from build123d import *

# Parameters (mm, degrees)
SKETCH_1_W               = 40
SKETCH_1_H               = 30
EXTRUDE_1_DEPTH          = 125
SKETCH_2_W               = 38
SKETCH_2_H               = 28
CUT_EXTRUDE_1_DEPTH      = 126
CUT_EXTRUDE_1_DEPTH_BACK = 126
SKETCH_3_R               = 2.025
CUT_EXTRUDE_2_DEPTH      = 1
CUT_EXTRUDE_2_DEPTH_BACK = 31
SKETCH_4_R               = 2.025
CUT_EXTRUDE_3_DEPTH      = 1
CUT_EXTRUDE_3_DEPTH_BACK = 31
CUT_EXTRUDE_4_DEPTH      = 1
CUT_EXTRUDE_4_DEPTH_BACK = 41
CUT_EXTRUDE_5_DEPTH      = 1
CUT_EXTRUDE_5_DEPTH_BACK = 31
CUT_EXTRUDE_6_DEPTH      = 1
CUT_EXTRUDE_6_DEPTH_BACK = 41


with BuildPart() as part:
    # 草图1 → 凸台-拉伸1 (new body, symmetric)
    with BuildSketch(Plane(origin=(0, 0, 0), x_dir=(1, 0, 0), z_dir=(0, 1, 0))):
        Rectangle(SKETCH_1_W, SKETCH_1_H)
    extrude(amount=EXTRUDE_1_DEPTH, both=True)

    # 草图2 → 切除-拉伸1 (cut, two sides)
    with BuildSketch(Plane(origin=(0, 0, 0), x_dir=(1, 0, 0), z_dir=(0, 1, 0))) as cut_extrude_1_sk:
        Rectangle(SKETCH_2_W, SKETCH_2_H)
    extrude(amount=CUT_EXTRUDE_1_DEPTH, mode=Mode.SUBTRACT)
    extrude(cut_extrude_1_sk.sketch, amount=-CUT_EXTRUDE_1_DEPTH_BACK, mode=Mode.SUBTRACT)

    # 草图3 → 切除-拉伸2 (cut, two sides)
    with BuildSketch(Plane.XY.offset(15)) as cut_extrude_2_sk:
        with Locations((0, -62.433034374)):
            Circle(SKETCH_3_R)
        with Locations((0, -93.433034374)):
            Circle(SKETCH_3_R)
        with Locations((0, -121)):
            Circle(SKETCH_3_R)
    extrude(amount=CUT_EXTRUDE_2_DEPTH, mode=Mode.SUBTRACT)
    extrude(cut_extrude_2_sk.sketch, amount=-CUT_EXTRUDE_2_DEPTH_BACK, mode=Mode.SUBTRACT)

    # 草图4 → 切除-拉伸3 (cut, two sides)
    with BuildSketch(Plane(origin=(0, 0, -15), x_dir=(-1, 0, 0), z_dir=(0, 0, -1))) as cut_extrude_3_sk:
        with Locations((0, 120)):
            Circle(SKETCH_4_R)
        with Locations((12.5, 95)):
            Circle(SKETCH_4_R)
        with Locations((-12.5, 95)):
            Circle(SKETCH_4_R)
    extrude(amount=CUT_EXTRUDE_3_DEPTH, mode=Mode.SUBTRACT)
    extrude(cut_extrude_3_sk.sketch, amount=-CUT_EXTRUDE_3_DEPTH_BACK, mode=Mode.SUBTRACT)

    # 草图5 → 切除-拉伸4 (cut, two sides)
    with BuildSketch(Plane(origin=(20, 0, 0), x_dir=(0, 0, -1), z_dir=(1, 0, 0))) as cut_extrude_4_sk:
        with BuildLine():
            Line((-8, -100), (-8, -80))
            ThreePointArc((-8, -80), (0, -72), (8, -80))
            Line((8, -80), (8, -100))
            ThreePointArc((8, -100), (0, -108), (-8, -100))
        make_face()
    extrude(amount=CUT_EXTRUDE_4_DEPTH, mode=Mode.SUBTRACT)
    extrude(cut_extrude_4_sk.sketch, amount=-CUT_EXTRUDE_4_DEPTH_BACK, mode=Mode.SUBTRACT)

    # 草图6 → 切除-拉伸5 (cut, two sides)
    with BuildSketch(Plane(origin=(0, 0, -15), x_dir=(-1, 0, 0), z_dir=(0, 0, -1))) as cut_extrude_5_sk:
        with BuildLine():
            Line((-5, 115.5), (5, 115.5))
            ThreePointArc((5, 115.5), (13, 107.5), (5, 99.5))
            Line((5, 99.5), (-5, 99.5))
            ThreePointArc((-5, 99.5), (-13, 107.5), (-5, 115.5))
        make_face()
    extrude(amount=CUT_EXTRUDE_5_DEPTH, mode=Mode.SUBTRACT)
    extrude(cut_extrude_5_sk.sketch, amount=-CUT_EXTRUDE_5_DEPTH_BACK, mode=Mode.SUBTRACT)

    # 草图7 → 切除-拉伸6 (cut, two sides)
    with BuildSketch(Plane(origin=(20, 0, 0), x_dir=(0, 0, -1), z_dir=(1, 0, 0))) as cut_extrude_6_sk:
        with BuildLine():
            Line((-6, 45), (-6, 75))
            ThreePointArc((-6, 75), (0, 81), (6, 75))
            Line((6, 75), (6, 45))
            ThreePointArc((6, 45), (0, 39), (-6, 45))
        make_face()
        with BuildLine():
            Line((-6, -30), (-6, 0))
            ThreePointArc((-6, 0), (0, 6), (6, 0))
            Line((6, 0), (6, -30))
            ThreePointArc((6, -30), (0, -36), (-6, -30))
        make_face()
    extrude(amount=CUT_EXTRUDE_6_DEPTH, mode=Mode.SUBTRACT)
    extrude(cut_extrude_6_sk.sketch, amount=-CUT_EXTRUDE_6_DEPTH_BACK, mode=Mode.SUBTRACT)


solid = part.part
Can you work these out from the model? Positions are in its coordinate system, mm. A direction names the side the tool comes from. Give positions to 0.01 mm unless a question says otherwise; leave off trailing zeros. Order: outer loops, then holes, each group sorted by start corner. A loop starts at its lowest first (then second) coordinate and runs counter-clockwise, first axis right, second up. Notation, with made-up numbers: M -37.75,45.25 L 8.25,45.25 A11 cw 8.25,50.25 Z; hole C 19.25,17 d7. An arc over 180 degrees is marked long. Use a Markdown table: item, result. Add a question column.
Item 1: For faces 1 (the flat face through (0, 2, -14)), 2 (the cylindrical face through (-12.998, 107.676, -14.507)), 3 (the cylindrical face through (-19.5, 6, 0.1)), which set-ups out of +Z, -Z, +X, -X, +Y, -Y let a thin tool reach every point of the face, with its end or its side?
Item 2: Suppose I cut it at B-B (z = -3.25). Count the separate pieces of the cut face and the enclosed holes in it, then the cut area to 3 significant figures.
Item 3: Suppose I cut it at A-A (z = 11.25). List the corners of the cut face in (x, y) for me, then the cut area to 3 significant figures.
Item 4: We'd pull the mould along X, two halves only. Please class faces 4 (the cylindrical face through (19.507, -72.002, 0.176)), 5 (the flat face through (20, 2, 7)), 6 (the cylindrical face through (12.998, 107.324, 14.493)): +X half, -X half, draft (parallel to the pull), parting line (faces both ways), or undercut.
Item 5: If I drill on L1, parallel to Y at x = 0, z = -14.7 (3 decimals); L2, parallel to Z at x = -10.5, y = -70; L3, parallel to X at y = -53, z = -12.25, over which ranges is the centre line in solid material (lowest first)? Write a range as [from, to].
Item 6: Will this pin go through, and if not, where does the flat tip stop? pin 1 (3.5 mm diameter, centred on x = -12.5, y = 95, fed in from -Z).
Answer sheet:
| question | item | result |
|---|---|---|
| 1 | face 1 | +Y, -Y |
| 1 | face 2 | +Z, -Z |
| 1 | face 3 | +X, -X |
| 2 | separate pieces | 8 |
| 2 | enclosed holes | 0 |
| 2 | area | 270 mm² |
| 3 | outline | M -20,-125 L -19,-125 L -19,125 L -20,125 Z; M 19,-125 L 20,-125 L 20,125 L 19,125 Z |
| 3 | area | 500 mm² |
| 4 | face 4 | draft |
| 4 | face 5 | +X half |
| 4 | face 6 | undercut |
| 5 | L1 | y = [-125, -123.025], [-118.975, -95.458], [-91.408, -64.458], [-60.408, 99.5], [115.5, 117.975], [122.025, 125] |
| 5 | L2 | z = [-15, -14], [14, 15] |
| 5 | L3 | x = [-20, -19], [19, 20] |
| 6 | pin 1 | passes through |
